Build history of the part. All positions in model axes, mm. Give positions to 0.01 mm unless a question says otherwise; leave off trailing zeros. Order: outer loops, then holes, each group sorted by start corner. A loop starts at its lowest first (then second) coordinate and runs counter-clockwise, first axis right, second up. Notation, with made-up numbers: (89, 34.5) - (93, 34.5) arc R19 cw to (93, 39.5) - close; hole circle Ø3 at (17, 7). An arc over 180 degrees is marked (long way). Use a Markdown table: item, result. Add a question column.
(1) Slice it at A-A (x = 5.08). Write the cut outline in (y, z), then the cut area to 3 significant figures.
(2) Slice it at B-B (y = 27.5). Write the cut outline in (x, z).
(3) Slice it at D-D (x = 18). Write the cut outline in (y, z).
(4) Slice it at C-C (z = -12). Write the cut outline in (x, y), then the cut area to 3 significant figures.
(5) Wall check: line 1 (Y direction, x = 5.08, z = 1.9); line 2 (Z direction, x = 4, y = 43.5); line 3 (X direction, y = 21, z = -2). Give the ranges that are in metal, low to high.
(6) Flat gauge pins, fed straight in: pin 1 (12 mm diameter, centred on x = 11, z = -0.5, fed in from +Y); pin 2 (1.4 mm diameter, centred on x = 1.5, y = -59, fed in from +Z); pin 3 (8 mm diameter, centred on y = -19.5, z = -9, fed in from +X); pin 4 (11 mm diameter, centred on x = 7.5, y = -64, fed in from +Z). Where does each tip first touch, or does it go through?
from build123d import *

# Parameters (mm, degrees)
F1_DEPTH  = 2.54
F3_DEPTH  = 7.62
F4_W      = 152.748324
F4_H      = 2.212828
F5_DEPTH  = 25.4
F6_R      = 1.577712
F7_DEPTH  = 4.293219
F8_W      = 152.748324
F8_H      = 2.120568
F9_DEPTH  = 1.778
F10_W     = 3.754646
F10_H     = 2.120568
F11_DEPTH = 1.778


with BuildPart() as f1:
    # F0 (on Right) → F1 (new body)
    with BuildSketch(Plane.YZ):
        Polygon((76.487139, 12.653703), (-58.410417, 12.653703), (-58.410417, 4.293219), (-76.261185, 4.293219), (-76.261185, -17.172892), (76.487139, -17.172892), align=None)
    extrude(amount=F1_DEPTH)

    # F2 (on face) → F3 (join)
    with BuildSketch(Plane.YZ.offset(2.54)):
        Polygon((-58.410417, 4.293219), (-76.261185, 4.293219), (-76.261185, 0), (-58.395639, 0), (-58.395639, 4.293219), align=None)
    extrude(amount=F3_DEPTH)

    # F4 (on face) → F5 (join)
    with BuildSketch(Plane.YZ.offset(2.54)):
        with Locations((0.112977, -16.066478)):
            Rectangle(F4_W, F4_H)
    extrude(amount=F5_DEPTH)

    # F6 (on face) → F7 (cut, through all)
    with BuildSketch(Plane.XY.offset(4.293219)):
        with Locations((5.08, -67.335801)):
            Circle(F6_R)
    extrude(amount=-F7_DEPTH, mode=Mode.SUBTRACT)

    # F8 (on face) → F9 (cut)
    with BuildSketch(Plane.YZ.offset(2.54)):
        with Locations((0.112977, -1.060284)):
            Rectangle(F8_W, F8_H)
    extrude(amount=-F9_DEPTH, mode=Mode.SUBTRACT)

    # F10 (on face) → F11 (join)
    with BuildSketch(Plane.YZ.offset(0.762)):
        with Locations((-24.277054, -1.060284)):
            Rectangle(F10_W, F10_H)
    extrude(amount=F11_DEPTH)


solid = f1.part
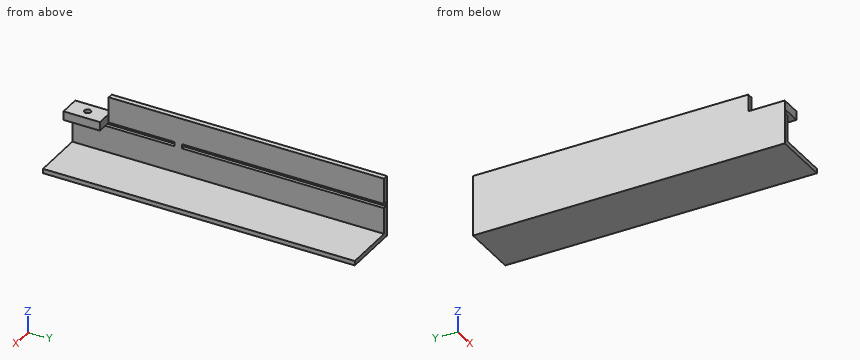
Solution:
| question | item | result |
|---|---|---|
| 1 | outline | (-76.26, -17.17) - (76.49, -17.17) - (76.49, -14.96) - (-76.26, -14.96) - close; (-76.26, 0) - (-68.91, 0) - (-68.91, 4.29) - (-76.26, 4.29) - close; (-65.76, 0) - (-58.4, 0) - (-58.4, 4.29) - (-65.76, 4.29) - close |
| 1 | area | 401 mm2 |
| 2 | outline | (0, -17.17) - (27.94, -17.17) - (27.94, -14.96) - (2.54, -14.96) - (2.54, -2.12) - (0.76, -2.12) - (0.76, 0) - (2.54, 0) - (2.54, 12.65) - (0, 12.65) - close |
| 3 | outline | (-76.26, -17.17) - (76.49, -17.17) - (76.49, -14.96) - (-76.26, -14.96) - close |
| 4 | outline | (0, -76.26) - (2.54, -76.26) - (2.54, 76.49) - (0, 76.49) - close |
| 4 | area | 388 mm2 |
| 5 | line 1 | -76.26 to -68.91, -65.76 to -58.4 |
| 5 | line 2 | -17.17 to -14.96 |
| 5 | line 3 | 0 to 0.76 |
| 6 | pin 1 | y = -58.4 |
| 6 | pin 2 | z = 12.65 |
| 6 | pin 3 | x = 2.54 |
| 6 | pin 4 | z = 4.29 |
